Autodesk Inventor part; units mm, degrees
ref_plane "YZ Plane" through (0, 0, 0) normal (1, 0, 0) x (0, 1, 0)
ref_plane "XZ Plane" through (0, 0, 0) normal (0, 1, 0) x (-1, 0, 0)
ref_plane "XY Plane" through (0, 0, 0) normal (0, 0, 1) x (1, 0, 0)
sketch "Sketch1" plane through (0, 0, 0) normal (0, 1, 0) x (-1, 0, 0)
  circle A0 centre (0, 0) radius 7.5
  line L0 (10, -6) -> (-10, -6)
  line L1 (-10, -6) -> (-10, 6)
  line L2 (-10, 6) -> (10, 6)
  line L3 (10, 6) -> (10, -6)
  line L4 (10, -6) -> (-10, 6) construction
  line L5 (-10, -6) -> (10, 6) construction
  point P0 (4.5, 6)
  point P1 (-4.5, 6)
  point P2 (-4.5, -6)
  point P3 (4.5, -6)
  dimension "d0" = 15
  dimension "d1" = 12
  dimension "d2" = 20
extrude "Extrusion1" add sketch "Sketch1" along normal blind 17.9 contours A0 L0 L2
sketch "Sketch2" plane through (0, 0, 0) normal (0, -1, 0) x (1, 0, 0)
  circle A0 centre (0, 0) radius 2.35
  dimension "d5" = 4.7
extrude "Extrusion2" add sketch "Sketch2" along normal blind 1.5
sketch "Sketch3" plane through (0, -1.5, 0) normal (0, -1, 0) x (1, 0, 0)
  circle A0 centre (0, 0) radius 0.8
  dimension "d8" = 1.6
extrude "Extrusion3" add sketch "Sketch3" along normal blind 5.5
sketch "Sketch4" plane through (0, 17.9, 0) normal (0, 1, 0) x (1, 0, 0)
  circle A0 centre (0, 0) radius 0.8
  circle A1 centre (0, 0) radius 2.5
  dimension "d11" = 5
extrude "Extrusion4" add sketch "Sketch4" along normal blind 0.7 contours A0 | A1
sketch "Sketch6" plane through (0, 17.9, 0) normal (0, 1, 0) x (1, 0, 0)
  line L0 (4.6211, -0.2655) -> (4.345, -0.3827)
  line L1 (4.345, -0.3827) -> (3.7589, 0.998)
  line L2 (3.7589, 0.998) -> (4.035, 1.1153)
  line L3 (4.035, 1.1153) -> (4.6211, -0.2655)
  line L4 (4.6211, -0.2655) -> (3.7589, 0.998) construction
  line L5 (4.345, -0.3827) -> (4.035, 1.1153) construction
  line L6 (-4.345, 0.3827) -> (-4.6211, 0.2655)
  line L7 (-4.6211, 0.2655) -> (-4.035, -1.1153)
  line L8 (-4.035, -1.1153) -> (-3.7589, -0.998)
  line L9 (-3.7589, -0.998) -> (-4.345, 0.3827)
  line L10 (-4.345, 0.3827) -> (-4.035, -1.1153) construction
  line L11 (-4.6211, 0.2655) -> (-3.7589, -0.998) construction
  point P0 (0, 0)
  point P1 (4.19, 0.3663)
  point P2 (-4.19, -0.3663)
  dimension "d26" = 0.3
  dimension "d27" = 1.5
  dimension "d28" = 0.3
  dimension "d29" = 1.5
  dimension "d30" = 4.19
  dimension "d31" = 4.19
  dimension "d32" = -0.3663
  dimension "d33" = -0.3663
extrude "Extrusion5" add sketch "Sketch6" along normal blind 2.15
sketch "Sketch7" plane through (0, 0, 0) normal (0, -1, 0) x (1, 0, 0)
  line L0 (-6.7346, -3.8882) -> (6.7346, 3.8882) construction
  circle A0 centre (-4.3301, -2.5) radius 1.1
  circle A1 centre (4.3301, 2.5) radius 1.1
  point P0 (0, 0)
  point P1 (0, 0)
  dimension "d36" = 2.2
  dimension "d37" = 2.2
  dimension "d38" = 5
  dimension "d39" = 5
extrude "Extrusion6" cut sketch "Sketch7" against normal blind 2.15
properties part number "Silnik"
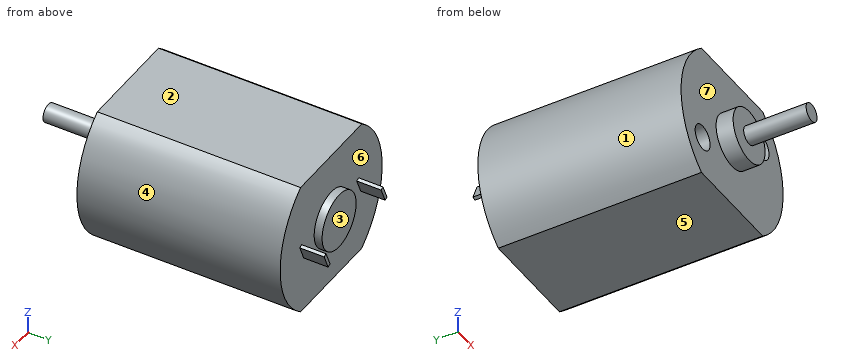
Could you check a few things on this model? Use its own coordinates, in mm. Face numbers are marked on the shaded views. A direction names the side the tool comes from. Round coordinates to 2 decimals unless told otherwise and drop trailing zeros. Order: outer loops, then holes, each group sorted by start corner. A loop starts at its lowest first (then second) coordinate and runs counter-clockwise, first axis right, second up.
Q1. Please list where these lines run through material, in increasing order: probe 1 along Y at (x, z) = (-6, 2.5); probe 2 along Y at (x, z) = (-4, -2); probe 3 along Z at (x, y) = (4.75, 3).
Geometry says:
probe 1: y = 0 to 17.9
probe 2: y = 2.15 to 17.9
probe 3: z = -5.8 to 5.8
Q2. Imagine slicing it at A-A, the plane x = 0. List the corners of the cut face in (y, z) for me.
Geometry says:
outline: (-7, -0.8) - (-1.5, -0.8) - (-1.5, -2.35) - (0, -2.35) - (0, -6) - (17.9, -6) - (17.9, -2.5) - (18.6, -2.5) - (18.6, 2.5) - (17.9, 2.5) - (17.9, 6) - (0, 6) - (0, 2.35) - (-1.5, 2.35) - (-1.5, 0.8) - (-7, 0.8) - close
Q3. Thinking about a two-plate mould opening in X: for the marked faces 1, 2, 3 and 4, which applies, released by +X, released by -X, zero draft, split by the parting line, or undercut?
Geometry says:
face 1: released by -X
face 2: zero draft
face 3: undercut
face 4: released by +X
Q4. Imagine slicing it at D-D, the plane y = 14.25. List the corners of the cut face in (x, z) for me.
Geometry says:
outline: (-4.5, -6) - (4.5, -6) arc R7.5 ccw to (4.5, 6) - (-4.5, 6) arc R7.5 ccw to start
Q5. Imagine slicing it at C-C, the plane z = 1.75. List the corners of the cut face in (x, y) for me.
Geometry says:
outline: (-7.29, 0) - (-1.57, 0) - (-1.57, -1.5) - (1.57, -1.5) - (1.57, 0) - (3.53, 0) - (3.53, 2.15) - (5.13, 2.15) - (5.13, 0) - (7.29, 0) - (7.29, 17.9) - (1.79, 17.9) - (1.79, 18.6) - (-1.79, 18.6) - (-1.79, 17.9) - (-7.29, 17.9) - close
Q6. I'm going to push flat-ended pins straight in: P1, Ø3.5, axis at x = -4.33, z = -2.5, coming from the -Y side; P2, Ø1.5, axis at x = 1, z = 0, coming from the +Y side; P3, Ø3.5, axis at x = -2.5, z = 1, coming from the -Y side. Where does each tip first touch, or does it pass through?
Geometry says:
P1: stops at y = 0
P2: stops at y = 18.6
P3: stops at y = -1.5
Q7. Which directions (+Z, -Z, +X, -X, +Y, -Y) give clear straight access to the entire face, cutting with the end or side of a thin tool? Please do the marked faces 5, 6 and 7.
Geometry says:
face 5: -Z, +X, -X, +Y, -Y
face 6: +Y
face 7: -Y
Q8. Imagine slicing it at B-B, the plane y = 1. List the corners of the cut face in (x, z) for me.
Geometry says:
outline: (-4.5, -6) - (4.5, -6) arc R7.5 ccw to (4.5, 6) - (-4.5, 6) arc R7.5 ccw to start; hole circle Ø2.2 at (-4.33, -2.5); hole circle Ø2.2 at (4.33, 2.5)
